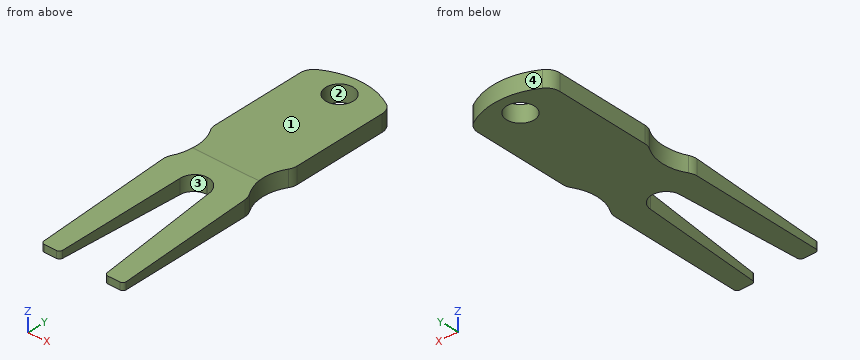
from build123d import *

# Parameters (mm, degrees)
F0_R        = 3.175
F1_DEPTH    = 3.81
F2_R        = 3.302
F3_T1_DEPTH = 7.6195000328
F3_T3_DEPTH = 7.3891966687
F5_DEPTH    = 3.811
F6_R        = 3.175
F8_DEPTH    = 18.797


# Not quite as in the source:
# - a fillet or chamfer that OpenCascade refuses, or shapes differently, is made with other operations: its cross-section is extruded or revolved along the edge and cut away or added


with BuildPart() as f1:
    # F0 (on Top) → F1 (new body)
    with BuildSketch(Plane.XY):
        with BuildLine():
            ThreePointArc((8.9284270597, -22.9513050998), (7.6006411438, -16.7271260659), (10.4890512239, -11.0561025874))
            ThreePointArc((10.4890512239, -11.0561025874), (0, 15.24), (-10.4890512239, -11.0561025874))
            ThreePointArc((-10.4890512239, -11.0561025874), (-7.6006411438, -16.7271260659), (-8.9284270597, -22.9513050998))
            ThreePointArc((-8.9284270597, -22.9513050998), (-9.2783523459, -23.7496251472), (-9.398, -24.6130178983))
            Line((-9.398, -24.6130178983), (-9.398, -55.5625))
            Line((-9.398, -55.5625), (-5.1562, -55.5625))
            Line((-5.1562, -55.5625), (-3.175, -23.8125))
            Line((-3.175, -23.8125), (3.175, -23.8125))
            Line((3.175, -23.8125), (5.1562, -55.5625))
            Line((5.1562, -55.5625), (9.398, -55.5625))
            Line((9.398, -55.5625), (9.398, -24.6130178983))
            ThreePointArc((9.398, -24.6130178983), (9.2783523459, -23.7496251472), (8.9284270597, -22.9513050998))
        make_face()
        with Locations((0, 9.921875)):
            Circle(F0_R, mode=Mode.SUBTRACT)
    extrude(amount=-F1_DEPTH)

    # F2
    f2_edges = [f1.edges().sort_by_distance(p)[0] for p in [
        (-3.175, -23.8125, -1.905),
        (3.175, -23.8125, -1.905),
    ]]
    fillet(f2_edges, radius=F2_R)

    # F3: fillet of radius 0.762 on 4 edges, made by hand

    # F3_s2 → F3_t1 (cut)
    with BuildSketch(Plane.XY.offset(-5.7147500164)):
        with BuildLine():
            ThreePointArc((8.6361, -55.5626), (9.1749153673, -55.3394153673), (9.3981, -54.8006))
            Line((9.3981, -54.8006), (9.41334, -54.8006))
            ThreePointArc((9.41334, -54.8006), (9.41324, -55.18155), (9.41324, -55.5625))
            Line((9.41324, -55.5625), (9.398, -55.57774))
            ThreePointArc((9.398, -55.57774), (9.01705, -55.57774), (8.6361, -55.57784))
            Line((8.6361, -55.57784), (8.6361, -55.5626))
        make_face()
        with BuildLine():
            ThreePointArc((-8.6361, -55.5626), (-9.1749153673, -55.3394153673), (-9.3981, -54.8006))
            Line((-9.3981, -54.8006), (-9.41334, -54.8006))
            ThreePointArc((-9.41334, -54.8006), (-9.41324, -55.18155), (-9.41324, -55.5625))
            Line((-9.41324, -55.5625), (-9.398, -55.57774))
            ThreePointArc((-9.398, -55.57774), (-9.01705, -55.57774), (-8.6361, -55.57784))
            Line((-8.6361, -55.57784), (-8.6361, -55.5626))
        make_face()
    extrude(amount=F3_T1_DEPTH, mode=Mode.SUBTRACT)

    # F3_s4 → F3_t3 (cut)
    with BuildSketch(Plane.XY.offset(-5.5995983343)):
        with BuildLine():
            ThreePointArc((-5.111518531, -54.8480564977), (-5.350272066, -55.3559403691), (-5.8720393267, -55.5626))
            Line((-5.8720393267, -55.5626), (-5.8720393267, -55.57784))
            ThreePointArc((-5.8720393267, -55.57784), (-5.5141196634, -55.57774), (-5.1562, -55.57774))
            Line((-5.1562, -55.57774), (-5.1409895841, -55.56344913))
            ThreePointArc((-5.1409895841, -55.56344913), (-5.1186987525, -55.2062242648), (-5.096308115, -54.8490056276))
            Line((-5.096308115, -54.8490056276), (-5.111518531, -54.8480564977))
        make_face()
        with BuildLine():
            ThreePointArc((5.111518531, -54.8480564977), (5.350272066, -55.3559403691), (5.8720393267, -55.5626))
            Line((5.8720393267, -55.5626), (5.8720393267, -55.57784))
            ThreePointArc((5.8720393267, -55.57784), (5.5141196634, -55.57774), (5.1562, -55.57774))
            Line((5.1562, -55.57774), (5.1409895841, -55.56344913))
            ThreePointArc((5.1409895841, -55.56344913), (5.1186987525, -55.2062242648), (5.096308115, -54.8490056276))
            Line((5.096308115, -54.8490056276), (5.111518531, -54.8480564977))
        make_face()
    extrude(amount=F3_T3_DEPTH, mode=Mode.SUBTRACT)

    # F4 (on face) → F5 (cut, through all)
    with BuildSketch(Plane.XY):
        Polygon((-9.398, -15.875), (-9.398, 17.78), (9.398, 17.78), (9.398, -15.875), (19.05, -15.875), (19.05, 20.32), (-19.05, 20.32), (-19.05, -15.875), align=None)
    extrude(amount=-F5_DEPTH, mode=Mode.SUBTRACT)

    # F6
    f6_edges = [f1.edges().sort_by_distance(p)[0] for p in [
        (9.398, 11.9973, -1.905),
        (-9.398, 11.9973, -1.905),
        (-9.398, -12.286952, -1.905),
        (9.398, -12.286952, -1.905),
    ]]
    fillet(f6_edges, radius=F6_R)

    # F7 (on face) → F8 (cut, through all)
    with BuildSketch(Plane.YZ.offset(9.398)):
        Polygon((-57.15, 0), (-57.15, -2.286), (-19.05, 0), align=None)
    extrude(amount=-F8_DEPTH, mode=Mode.SUBTRACT)


solid = f1.part
Verification items for the finished model (mm, model axes). Face numbers are marked on the shaded views. Coordinates: 2 decimals unless noted, no trailing zeros. Order: outer loops, then holes, each group sorted by start corner. A loop starts at its lowest first (then second) coordinate and runs counter-clockwise, first axis right, second up.
Item 1: Material ranges on L1, parallel to Y at x = 0, z = -2.1; L2, parallel to Z at x = -5, y = -27; L3, parallel to Y at x = 2.5, z = -3, recorded low to high.
Filled in:
L1: y = -23.81 to 6.75, 13.1 to 15.24
L2: z = -3.81 to -0.48
L3: y = -24.88 to 7.96, 11.88 to 15.03
Item 2: Depth check by flat-ended pin: pin 1 (1 mm diameter, centred on x = 4.5, z = -1, fed in from +Y). Enter the tip coordinate at first touch or a pass-through.
Filled in:
pin 1: stops at y = 14.71
Item 3: Section check A-A, the plane y = -41. Enter the section's corners in (x, z), then the cut area to 3 significant figures.
Filled in:
outline: (-9.4, -3.81) - (-4.25, -3.81) - (-4.25, -1.32) - (-9.4, -1.32) - close; (4.25, -3.81) - (9.4, -3.81) - (9.4, -1.32) - (4.25, -1.32) - close
area: 25.7 mm2
Item 4: Section check B-B, the plane x = -2.5. Enter the section's corners in (y, z).
Filled in:
outline: (-24.88, -3.81) - (7.96, -3.81) - (7.96, 0) - (-19.05, 0) - (-24.88, -0.35) - close; (11.88, -3.81) - (15.03, -3.81) - (15.03, 0) - (11.88, 0) - close
Item 5: Section check D-D, the plane y = -14.5. Enter the section's corners in (x, z).
Filled in:
outline: (-8.17, -3.81) - (8.17, -3.81) - (8.17, 0) - (-8.17, 0) - close
Item 6: Release check for a two-part mould opening along X. For the marked faces 1, 2, 3 and 4 record: +X half, -X half, draft (parallel to the pull), parting line (faces both ways), or undercut.
Filled in:
face 1: draft
face 2: undercut
face 3: undercut
face 4: parting line
